Answer from the drawing. Dimensions are ordinates in mm from the lowest x, y and z of the part. Coordinates: 2 decimals unless noted, no trailing zeros. Write each loop counter-clockwise with the first axis right and the second up, starting at its lowest first coordinate (ties: lowest second). Pieces come first, ordered by that corner, then holes.
(1) The part is cut by section B-B on z = 1. Determine the outline of the cut face in (x, y), plus the area to 3 significant figures.
(2) The part is cut by section C-C on y = 0.35. Determine the outline of the cut face in (x, z).
(3) The part is cut by section A-A on x = 1. Determine the outline of the cut face in (y, z), plus the area to 3 significant figures.
(4) For a pull along X with two mould halves and no side action, classify the marked faces 1, 2, 3 and 4 as +X half, -X half, draft (parallel to the pull), parting line (faces both ways), or undercut.
(5) Straight lines are drawn through the part: line 1 (X direction, y = 0.55, z = 1.05); line 2 (Z direction, x = 1, y = 1.4); line 3 (X direction, y = 0.65, z = 0.7). For each, find the intervals that lie inside material, in ascending order.
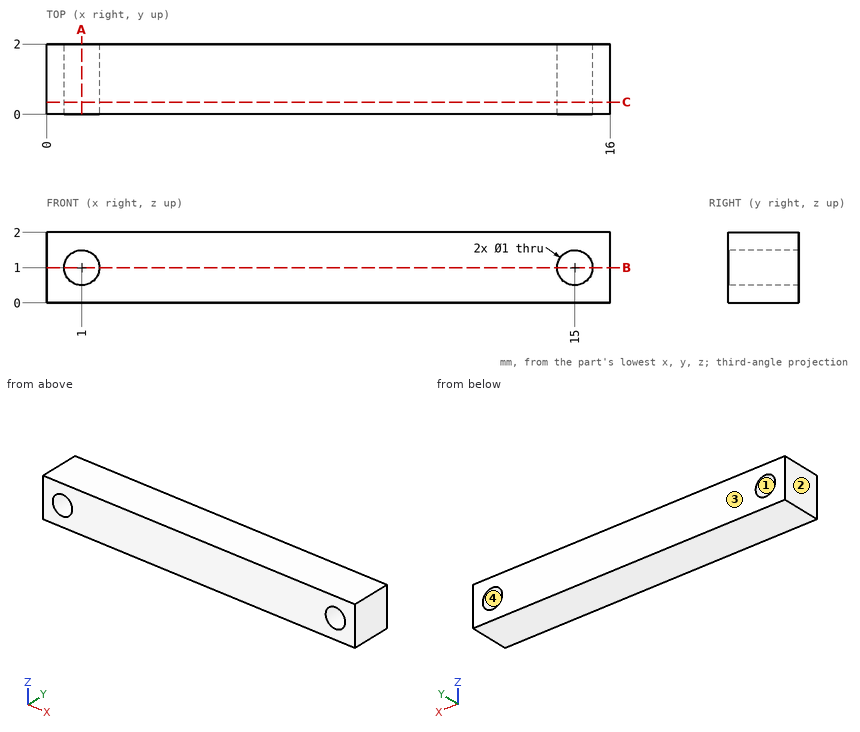
Model answer:
1. outline: (0, 0) - (0.5, 0) - (0.5, 2) - (0, 2) - close; (1.5, 0) - (14.5, 0) - (14.5, 2) - (1.5, 2) - close; (15.5, 0) - (16, 0) - (16, 2) - (15.5, 2) - close
1. area: 28.0 mm2
2. outline: (0, 0) - (16, 0) - (16, 2) - (0, 2) - close; hole circle Ø1 at (1, 1); hole circle Ø1 at (15, 1)
3. outline: (0, 0) - (2, 0) - (2, 0.5) - (0, 0.5) - close; (0, 1.5) - (2, 1.5) - (2, 2) - (0, 2) - close
3. area: 2.00 mm2
4. face 1: undercut
4. face 2: -X half
4. face 3: draft
4. face 4: undercut
5. line 1: x = 0 to 0.5, 1.5 to 14.5, 15.5 to 16
5. line 2: z = 0 to 0.5, 1.5 to 2
5. line 3: x = 0 to 0.6, 1.4 to 14.6, 15.4 to 16
